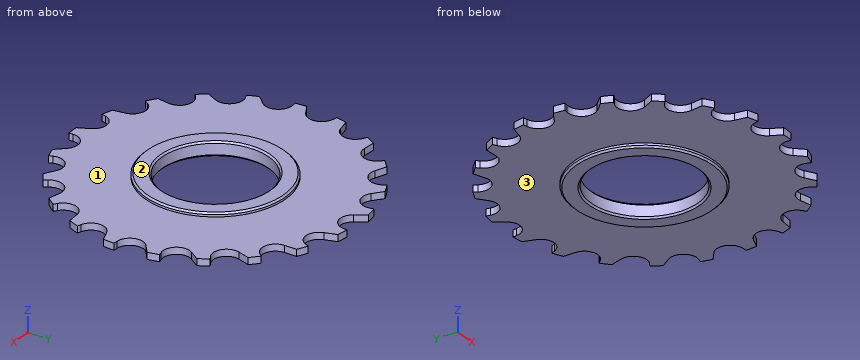
```python
from build123d import *

# Parameters (mm, degrees)
ESQUISSE1_R                  = 42.75
EXTRUSION1_DEPTH             = 1
ENL_V_MAT_EXTRU_1_DEPTH      = 2
R_P_TITION_CIRCULAIRE1_COUNT = 21
ESQUISSE3_R                  = 21
EXTRUSION2_DEPTH             = 2.125
ESQUISSE4_R                  = 16
ENL_V_MAT_EXTRU_2_DEPTH      = 3.125
ENL_V_MAT_EXTRU_2_DEPTH_BACK = 3.125
CHANFREIN1_SIZE              = 0.5


with BuildPart() as part:
    # Esquisse1 → Extrusion1 (new body, symmetric)
    with BuildSketch(Plane.XY):
        Circle(ESQUISSE1_R)
    extrude(amount=EXTRUSION1_DEPTH, both=True)

    # Esquisse2 → Enlèv. mat.-Extru.1 (cut, symmetric)
    with BuildSketch(Plane.XY):
        with BuildLine():
            Line((-5.348139413, 42.414147461), (-3.276608177, 39.455694255))
            ThreePointArc((-3.276608177, 39.455694255), (1.018480402, 37.881835362), (3.981599184, 41.366766467))
            Line((3.981599184, 41.366766467), (4.095808383, 42.553341275))
            ThreePointArc((4.095808383, 42.553341275), (-0.630021414, 42.745357327), (-5.348139413, 42.414147461))
        make_face()
    enl_v_mat_extru_1 = extrude(amount=ENL_V_MAT_EXTRU_1_DEPTH, both=True, mode=Mode.SUBTRACT)

    # Répétition circulaire1: Enlèv. mat.-Extru.1 ×21 about axis
    r_p_tition_circulaire1_axis = Axis((0, 0, 0), (0, 0, 1))
    for i in range(1, R_P_TITION_CIRCULAIRE1_COUNT):
        add(enl_v_mat_extru_1.rotate(r_p_tition_circulaire1_axis, i * 360 / R_P_TITION_CIRCULAIRE1_COUNT), mode=Mode.SUBTRACT)

    # Esquisse3 → Extrusion2 (add, symmetric)
    with BuildSketch(Plane.XY):
        Circle(ESQUISSE3_R)
    extrude(amount=EXTRUSION2_DEPTH, both=True)

    # Esquisse4 → Enlèv. mat.-Extru.2 (cut, two sides)
    with BuildSketch(Plane.XY) as enl_v_mat_extru_2_sk:
        Circle(ESQUISSE4_R)
    extrude(amount=ENL_V_MAT_EXTRU_2_DEPTH, mode=Mode.SUBTRACT)
    extrude(enl_v_mat_extru_2_sk.sketch, amount=-ENL_V_MAT_EXTRU_2_DEPTH_BACK, mode=Mode.SUBTRACT)

    # Chanfrein1
    chanfrein1_edges = [part.edges().sort_by_distance(p)[0] for p in [
        (-21, 0, -2.125),
        (-21, 0, 2.125),
        (-16, 0, -2.125),
        (-16, 0, 2.125),
    ]]
    chamfer(chanfrein1_edges, length=CHANFREIN1_SIZE)


solid = part.part
```
Input: part model. Units: mm. Frame: model coordinates. Face numbers are marked on the shaded views. A direction names the side the tool comes from. Round coordinates to 2 decimals unless told otherwise and drop trailing zeros. Loops run counter-clockwise (first coordinate to the right, second up) from the corner with the lowest first, then second, coordinate; pieces in that order, holes last. Notation, with made-up numbers: (78, -20) -> (123, -20) arc R19 ccw to (123, -8) -> close; hole circle Ø5 at (8, -39). An arc over 180 degrees is marked (long way). Use one line per item in the form item = value. Start each with the question number.
Item 1: Set-up query: the marked faces 1, 2 and 3. Return all of +Z, -Z, +X, -X, +Y, -Y with unobstructed straight access to the full face (end or side cutting, diameter ignored); none if empty.
Item 2: Contact query for flat-ended pins moving along their axis: pin 1 Ø1.5 at (x, y) = (-30.5, 27.5) entering from -Z; pin 2 Ø1.5 at (x, z) = (-32, -1.5) entering from +Y; pin 3 Ø5 at (x, y) = (18, 23) entering from +Z; pin 4 Ø6 at (x, y) = (14.5, 34) entering from -Z. Output: stop coordinate, or through.
Item 3: Material intervals for L1, parallel to Y at x = 0, z = -0.1; L2, parallel to Y at x = -30, z = 0.7; L3, parallel to X at y = 2.5, z = -1.75, sorted ascending. Write a range as from..to.
Item 4: Section query A-A on x = 0. Return the cut outline in (y, z) (3 decimals).
Ans:
q1.face_1 = +Z
q1.face_2 = +Z, +X, -X, +Y, -Y
q1.face_3 = -Z
q2.pin_1 = through
q2.pin_2 = 22.22
q2.pin_3 = 1
q2.pin_4 = -1
q3.L1 = -42.75..-16, 16..37.75
q3.L2 = -26.94..23.03, 29.04..30.46
q3.L3 = -20.72..-15.93, 15.93..20.72
q4.outline = (-42.75, -1) -> (-21, -1) -> (-21, -1.625) -> (-20.5, -2.125) -> (-16.5, -2.125) -> (-16, -1.625) -> (-16, 1.625) -> (-16.5, 2.125) -> (-20.5, 2.125) -> (-21, 1.625) -> (-21, 1) -> (-42.75, 1) -> close; (16, -1.625) -> (16.5, -2.125) -> (20.5, -2.125) -> (21, -1.625) -> (21, -1) -> (37.75, -1) -> (37.75, 1) -> (21, 1) -> (21, 1.625) -> (20.5, 2.125) -> (16.5, 2.125) -> (16, 1.625) -> close
